```python
from build123d import *

# Parameters (mm, degrees)
F0_W     = 10
F0_H     = 10
F1_DEPTH = 5
F3_DEPTH = 10
F2_W     = 4.5
F2_H     = 6.5
F4_DEPTH = 2.5
F6_DEPTH = 2.5
F7_W     = 4.5
F7_H     = 1.5
F8_DEPTH = 1.5


with BuildPart() as f1:
    # F0 (on Top) → F1 (new body)
    with BuildSketch(Plane.XY):
        with Locations((0, -1.2614674985)):
            Rectangle(F0_W, F0_H)
    extrude(amount=F1_DEPTH)

    # F3 (add): a face of the model
    f3_faces = [f1.faces().sort_by_distance(p)[0] for p in [
        (0, -6.2614674985, 2.5),
    ]]
    extrude(f3_faces, amount=F3_DEPTH)

    # F2 (on face) → F4 (cut)
    with BuildSketch(Plane.XY.offset(5)):
        with Locations((0, -2.2614674985)):
            Rectangle(F2_W, F2_H)
    extrude(amount=-F4_DEPTH, mode=Mode.SUBTRACT)

    # F5 (on face) → F6 (cut)
    with BuildSketch(Plane.XY.offset(5)):
        Polygon((-4, -7.5114674985), (0, -14.4396707288), (4, -7.5114674985), align=None)
    extrude(amount=-F6_DEPTH, mode=Mode.SUBTRACT)

    # F7 (on face) → F8 (join)
    with BuildSketch(Plane.XY.offset(2.5)):
        with Locations((0, -2.2614674985)):
            Rectangle(F7_W, F7_H)
    extrude(amount=F8_DEPTH)


solid = f1.part
```
The listing builds one solid part. Answer for the finished solid, in the listing's coordinates (mm). A direction names the side the tool comes from. Give positions to 0.01 mm unless a question says otherwise; leave off trailing zeros. Loops run counter-clockwise (first coordinate to the right, second up) from the corner with the lowest first, then second, coordinate; pieces in that order, holes last. Notation, with made-up numbers: (46, 21.5) - (93, 21.5) arc R24 cw to (93, 42.5) - close; hole circle Ø4 at (-14, 65.5). An arc over 180 degrees is marked (long way). Answer as CSV lines item,"result". Start each with the question number.
Item 1: A cutting plane is placed at A-A on z = 3.2. Determine the outline of the cut face in (x, y), then the cut area to 3 significant figures.
Item 2: A cutting plane is placed at D-D on x = 2.5. Determine the outline of the cut face in (y, z), then the cut area to 3 significant figures.
Item 3: A cutting plane is placed at B-B on y = -0.75. Determine the outline of the cut face in (x, z).
Item 4: Find the intervals of material crossed by line 1 (Y direction, x = -1, z = 3.55); line 2 (X direction, y = -8.25, z = 3.3); line 3 (Y direction, x = 2, z = 3.8), in increasing order. Write a range as from..to.
Item 5: For faces 1 (the face through (-2.028, -10.927, 3.768)), 2 (the face through (-5, -6, 2)), determine the directions among +Z, -Z, +X, -X, +Y, -Y from which every point of the face is accessible in a straight line to the end or side of a thin tool.
Item 6: A cutting plane is placed at C-C on z = 4.6. Determine the outline of the cut face in (x, y).
Item 7: The mould has two halves that part along X. Classify faces 3 (the face through (0, 3.739, 2)), 4 (the face through (0, -7.511, 4)), 5 (the face through (5, -6, 2)): +X half, -X half, draft (parallel to the pull), parting line (faces both ways), or undercut.
Item 8: This flat-tipped pin is pushed along its axis until it touches: pin 1 (1 mm diameter, centred on x = -4, y = -12, fed in from -Z). Where does it stop, or does it pass through?
Found:
1,outline,"(-5, -16.26) - (5, -16.26) - (5, 3.74) - (-5, 3.74) - close; hole (-4, -7.51) - (0, -14.44) - (4, -7.51) - close; hole (-2.25, -5.51) - (2.25, -5.51) - (2.25, -3.01) - (-2.25, -3.01) - close; hole (-2.25, -1.51) - (2.25, -1.51) - (2.25, 0.99) - (-2.25, 0.99) - close"
1,area,"150 mm^2"
2,outline,"(-16.26, 0) - (3.74, 0) - (3.74, 5) - (-7.51, 5) - (-7.51, 2.5) - (-10.11, 2.5) - (-10.11, 5) - (-16.26, 5) - close"
2,area,"93.5 mm^2"
3,outline,"(-5, 0) - (5, 0) - (5, 5) - (2.25, 5) - (2.25, 2.5) - (-2.25, 2.5) - (-2.25, 5) - (-5, 5) - close"
4,line 1,"y = -16.26..-12.71, -7.51..-5.51, -3.01..-1.51, 0.99..3.74"
4,line 2,"x = -5..-3.57, 3.57..5"
4,line 3,"y = -16.26..-10.98, -7.51..-5.51, -3.01..-1.51, 0.99..3.74"
5,face 1,"+Z"
5,face 2,"+Z, -Z, -X, +Y, -Y"
6,outline,"(-5, -16.26) - (5, -16.26) - (5, 3.74) - (-5, 3.74) - close; hole (-4, -7.51) - (0, -14.44) - (4, -7.51) - close; hole (-2.25, -5.51) - (2.25, -5.51) - (2.25, 0.99) - (-2.25, 0.99) - close"
7,face 3,"draft"
7,face 4,"undercut"
7,face 5,"+X half"
8,pin 1,"stops at z = 0"
